Design review of the part built by this model. Coordinates are the model's own, in mm. A direction names the side the tool comes from. Round coordinates to 2 decimals unless told otherwise and drop trailing zeros. Order: outer loops, then holes, each group sorted by start corner. A loop starts at its lowest first (then second) coordinate and runs counter-clockwise, first axis right, second up. Notation, with made-up numbers: (17, -39) - (27, -39) arc R15 cw to (27, -29) - close; hole circle Ø7 at (-0.5, -32). An arc over 180 degrees is marked (long way). Write item = value, one per line.
from build123d import *

# Parameters (mm, degrees)
SKETCH_1_R           = 2
EXTRUDE_1_DEPTH      = 7.5
EXTRUDE_2_DEPTH      = 10
EXTRUDE_2_DEPTH_BACK = 1.5
SKETCH_2_R           = 2.5
SKETCH_5_R           = 3.1
CUT_EXTRUDE_1_DEPTH  = 4


with BuildPart() as part:
    # 草圖1 → 填料-伸長1 (new body)
    with BuildSketch(Plane.XY):
        with BuildLine():
            Line((-10, 5), (10, 5))
            ThreePointArc((10, 5), (15, 0), (10, -5))
            Line((10, -5), (-10, -5))
            ThreePointArc((-10, -5), (-15, 0), (-10, 5))
        make_face()
        with Locations((-10, 0)):
            Circle(SKETCH_1_R, mode=Mode.SUBTRACT)
        with Locations((10, 0)):
            Circle(SKETCH_1_R, mode=Mode.SUBTRACT)
    extrude(amount=EXTRUDE_1_DEPTH)

    # 草圖2 → 填料-伸長2 (add, two sides: drawn at the far end of the back side and taken through both)
    with BuildSketch(Plane.XY.offset(7.5).offset(-EXTRUDE_2_DEPTH_BACK)):
        with Locations((7.5, 0)):
            Circle(SKETCH_2_R)
    extrude(amount=EXTRUDE_2_DEPTH + EXTRUDE_2_DEPTH_BACK)

    # 草圖5 → 除料-伸長1 (cut)
    with BuildSketch(Plane(origin=(0, 0, 0), x_dir=(-1, 0, 0), z_dir=(0, 0, -1))):
        with Locations((-10, 0)):
            Circle(SKETCH_5_R)
        Polygon((5.882234711, -2.799315774), (9.115395929, -2.800683725), (10.733161218, -0.001367951), (9.117765289, 2.799315774), (5.884604071, 2.800683725), (4.266838782, 0.001367951), align=None)
    extrude(amount=-CUT_EXTRUDE_1_DEPTH, mode=Mode.SUBTRACT)


solid = part.part
Item 1: Take a section at A-A, the plane z = 2. State the section outline as (x, y) points, and give its area (3 significant figures).
Data:
outline = (-10, -5) - (10, -5) arc R5 ccw to (10, 5) - (-10, 5) arc R5 ccw to start; hole (-9.6, -1.96) - (-9.12, -2.8) - (-5.88, -2.8) - (-4.27, 0) - (-5.88, 2.8) - (-9.12, 2.8) - (-9.6, 1.96) arc R2 ccw (long way) to start; hole circle Ø6.2 at (10, 0)
area = 216 mm2
Item 2: Take a section at D-D, the plane z = 9.75. State the section outline as (x, y) points.
Data:
outline = circle Ø5 at (7.5, 0)
Item 3: For faces 1 (the face through (0, 5, 4)), 2 (the face through (9.885, 0.751, 11.67)), 3 (the face through (-7, 0, 4)), list the 3-axis set-ups (+Z, -Z, +X, -X, +Y, -Y) from which the entire face can be reached by the end or side of a thin tool; tool diameter is ignored.
Data:
face_1 = +Z, -Z, +X, -X, +Y
face_2 = +Z
face_3 = -Z
Item 4: The part is to be moulded in two halves that separate along X. For faces 4 (the face through (0, -5, 4)), 5 (the face through (13.1, 0.1, 2)), 6 (the face through (-15, 0, 4)), say which applies: +X half, -X half, draft (parallel to the pull), parting line (faces both ways), or undercut.
Data:
face_4 = draft
face_5 = undercut
face_6 = -X half
Item 5: For line 1 along X through (y, z) = (0, 4.8); line 2 along Y through (x, z) = (-10, 3); line 3 along X through (y, z) = (0, 6.7), list the stretches that pass through material, from the lowest coordinate up. Write a range as [from, to].
Data:
line_1 = [-15, -12], [-8, 8], [12, 15]
line_2 = [-5, -2], [2, 5]
line_3 = [-15, -12], [-8, 10], [12, 15]
Item 6: Take a section at B-B, the plane x = -11.25. State the section outline as (y, z) points, and give its area (3 significant figures).
Data:
outline = (-4.84, 0) - (-1.56, 0) - (-1.56, 7.5) - (-4.84, 7.5) - close; (1.56, 0) - (4.84, 0) - (4.84, 7.5) - (1.56, 7.5) - close
area = 49.2 mm2
Item 7: Insertion check: P1, Ø5, axis at x = -1.5, y = 0, coming from the +Z side; P2, Ø3, axis at x = 10.5, y = 0.5, coming from the -Z side; P3, Ø1.5, axis at y = 3, z = 2.5, coming from the +X side. Each pin has a flat end and moves straight along its axis. Give the tip position at first contact, or say it passes through.
Data:
P1 = 7.5
P2 = 4
P3 = 14.47
Item 8: Take a section at C-C, the plane x = 7.5. State the section outline as (y, z) points.
Data:
outline = (-5, 0) - (-1.83, 0) - (-1.83, 4) - (1.83, 4) - (1.83, 0) - (5, 0) - (5, 7.5) - (2.5, 7.5) - (2.5, 17.5) - (-2.5, 17.5) - (-2.5, 7.5) - (-5, 7.5) - close
